Source: three-view drawing plus pictorial views. Frame: mm from the lowest corner of the part. Round coordinates to 2 decimals unless told otherwise and drop trailing zeros. Loops run counter-clockwise (first coordinate to the right, second up) from the corner with the lowest first, then second, coordinate; pieces in that order, holes last. Notation, with made-up numbers: M 83,-16 L 87,-16 A16 ccw 87,-4 Z; hole C 6,76.5 d11. An arc over 180 degrees is marked long. Answer as a JSON object with one key per item and string values.
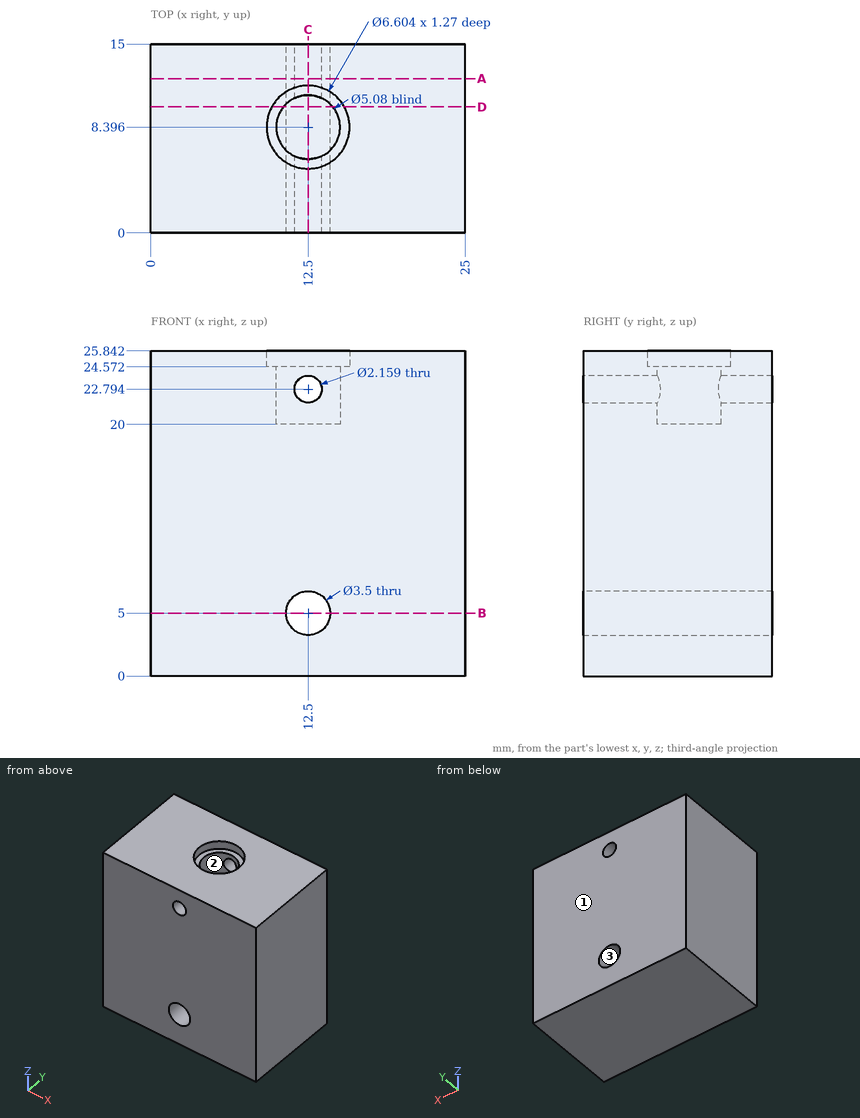
1) Cut plane B-B on z = 5. Return the cut outline in (x, y).
Geometry results:
{"outline": "M 0,0 L 10.75,0 L 10.75,15 L 0,15 Z; M 14.25,0 L 25,0 L 25,15 L 14.25,15 Z"}
2) Pull-direction query (Y, two-part tool) for the marked faces 1, 2 and 3; classes: +Y half, -Y half, draft (parallel to the pull), parting line (faces both ways), or undercut.
Geometry results:
{"face 1": "+Y half", "face 2": "undercut", "face 3": "draft"}
3) First-contact query: pin 1 (3 mm diameter, centred on x = 12.5, z = 5, fed in from -Y); pin 2 (6.5 mm diameter, centred on x = 12.5, y = 8.396, fed in from +Z). Flat tips, straight axial feed; report the tip coordinate or a pass-through.
Geometry results:
{"pin 1": "through", "pin 2": "z = 24.57"}
4) Cut plane C-C on x = 12.5. Return the cut outline in (y, z).
Geometry results:
{"outline": "M 0,0 L 15,0 L 15,3.25 L 0,3.25 Z; M 0,6.75 L 15,6.75 L 15,21.71 L 10.94,21.71 L 10.94,20 L 5.86,20 L 5.86,21.71 L 0,21.71 Z; M 0,23.87 L 5.86,23.87 L 5.86,24.57 L 5.09,24.57 L 5.09,25.84 L 0,25.84 Z; M 10.94,23.87 L 15,23.87 L 15,25.84 L 11.7,25.84 L 11.7,24.57 L 10.94,24.57 Z"}
5) Cut plane A-A on y = 12.25. Return the cut outline in (x, z).
Geometry results:
{"outline": "M 0,0 L 25,0 L 25,25.84 L 0,25.84 Z; hole C 12.5,5 d3.5; hole C 12.5,22.79 d2.16"}
6) Line query: probe 1 along Z at (x, y) = (12.5, 13.75); probe 2 along X at (y, z) = (5.25, 22.75); probe 3 along X at (y, z) = (11.75, 5). Output: solid intervals per line, ascending.
Geometry results:
{"probe 1": "0 to 3.25, 6.75 to 21.71, 23.87 to 25.84", "probe 2": "0 to 11.42, 13.58 to 25", "probe 3": "0 to 10.75, 14.25 to 25"}
7) Cut plane D-D on y = 10. Return the cut outline in (x, z).
Geometry results:
{"outline": "M 0,0 L 25,0 L 25,25.84 L 15.39,25.84 L 15.39,24.57 L 14.47,24.57 L 14.47,20 L 10.53,20 L 10.53,24.57 L 9.61,24.57 L 9.61,25.84 L 0,25.84 Z; hole C 12.5,5 d3.5"}
